```python
from build123d import *

# Parameters (mm, degrees)
SKETCH3_W           = 214
SKETCH3_H           = 93.282032303
BOSS_EXTRUDE1_DEPTH = 12.7
SKETCH2_R           = 9
CUT_EXTRUDE1_DEPTH  = 10
SKETCH5_R           = 7
CUT_EXTRUDE2_DEPTH  = 10


with BuildPart() as part:
    # Sketch3 → Boss-Extrude1 (new body)
    with BuildSketch(Plane(origin=(0, 0, 0), x_dir=(1, 0, 0), z_dir=(0, 1, 0))):
        with Locations((95, 34.641016152)):
            Rectangle(SKETCH3_W, SKETCH3_H)
    extrude(amount=BOSS_EXTRUDE1_DEPTH)

    # Sketch2 → Cut-Extrude1 (cut)
    with BuildSketch(Plane(origin=(0, 0, 0), x_dir=(1, 0, 0), z_dir=(0, 1, 0))):
        Circle(SKETCH2_R)
        with Locations((20, 0)):
            Circle(SKETCH2_R)
        with Locations((40, 0)):
            Circle(SKETCH2_R)
        with Locations((60, 0)):
            Circle(SKETCH2_R)
        with Locations((80, 0)):
            Circle(SKETCH2_R)
        with Locations((100, 0)):
            Circle(SKETCH2_R)
        with Locations((120, 0)):
            Circle(SKETCH2_R)
        with Locations((140, 0)):
            Circle(SKETCH2_R)
        with Locations((160, 0)):
            Circle(SKETCH2_R)
        with Locations((180, 0)):
            Circle(SKETCH2_R)
        with Locations((10, 17.320508076)):
            Circle(SKETCH2_R)
        with Locations((30, 17.320508076)):
            Circle(SKETCH2_R)
        with Locations((50, 17.320508076)):
            Circle(SKETCH2_R)
        with Locations((70, 17.320508076)):
            Circle(SKETCH2_R)
        with Locations((90, 17.320508076)):
            Circle(SKETCH2_R)
        with Locations((110, 17.320508076)):
            Circle(SKETCH2_R)
        with Locations((130, 17.320508076)):
            Circle(SKETCH2_R)
        with Locations((150, 17.320508076)):
            Circle(SKETCH2_R)
        with Locations((170, 17.320508076)):
            Circle(SKETCH2_R)
        with Locations((190, 17.320508076)):
            Circle(SKETCH2_R)
        with Locations((0, 34.641016151)):
            Circle(SKETCH2_R)
        with Locations((20, 34.641016151)):
            Circle(SKETCH2_R)
        with Locations((40, 34.641016151)):
            Circle(SKETCH2_R)
        with Locations((60, 34.641016151)):
            Circle(SKETCH2_R)
        with Locations((80, 34.641016151)):
            Circle(SKETCH2_R)
        with Locations((100, 34.641016151)):
            Circle(SKETCH2_R)
        with Locations((120, 34.641016151)):
            Circle(SKETCH2_R)
        with Locations((140, 34.641016151)):
            Circle(SKETCH2_R)
        with Locations((160, 34.641016151)):
            Circle(SKETCH2_R)
        with Locations((180, 34.641016151)):
            Circle(SKETCH2_R)
        with Locations((10, 51.961524227)):
            Circle(SKETCH2_R)
        with Locations((30, 51.961524227)):
            Circle(SKETCH2_R)
        with Locations((50, 51.961524227)):
            Circle(SKETCH2_R)
        with Locations((70, 51.961524227)):
            Circle(SKETCH2_R)
        with Locations((90, 51.961524227)):
            Circle(SKETCH2_R)
        with Locations((110, 51.961524227)):
            Circle(SKETCH2_R)
        with Locations((130, 51.961524227)):
            Circle(SKETCH2_R)
        with Locations((150, 51.961524227)):
            Circle(SKETCH2_R)
        with Locations((170, 51.961524227)):
            Circle(SKETCH2_R)
        with Locations((190, 51.961524227)):
            Circle(SKETCH2_R)
        with Locations((0, 69.282032303)):
            Circle(SKETCH2_R)
        with Locations((20, 69.282032303)):
            Circle(SKETCH2_R)
        with Locations((40, 69.282032303)):
            Circle(SKETCH2_R)
        with Locations((60, 69.282032303)):
            Circle(SKETCH2_R)
        with Locations((80, 69.282032303)):
            Circle(SKETCH2_R)
        with Locations((100, 69.282032303)):
            Circle(SKETCH2_R)
        with Locations((120, 69.282032303)):
            Circle(SKETCH2_R)
        with Locations((140, 69.282032303)):
            Circle(SKETCH2_R)
        with Locations((160, 69.282032303)):
            Circle(SKETCH2_R)
        with Locations((180, 69.282032303)):
            Circle(SKETCH2_R)
    extrude(amount=CUT_EXTRUDE1_DEPTH, mode=Mode.SUBTRACT)

    # Sketch5 → Cut-Extrude2 (cut)
    with BuildSketch(Plane.XZ.offset(-10)):
        Circle(SKETCH5_R)
        with Locations((20, 0)):
            Circle(SKETCH5_R)
        with Locations((40, 0)):
            Circle(SKETCH5_R)
        with Locations((80, 0)):
            Circle(SKETCH5_R)
        with Locations((60, 0)):
            Circle(SKETCH5_R)
        with Locations((100, 0)):
            Circle(SKETCH5_R)
        with Locations((120, 0)):
            Circle(SKETCH5_R)
        with Locations((140, 0)):
            Circle(SKETCH5_R)
        with Locations((160, 0)):
            Circle(SKETCH5_R)
        with Locations((180, 0)):
            Circle(SKETCH5_R)
        with Locations((190, -17.320508076)):
            Circle(SKETCH5_R)
        with Locations((170, -17.320508076)):
            Circle(SKETCH5_R)
        with Locations((150, -17.320508076)):
            Circle(SKETCH5_R)
        with Locations((130, -17.320508076)):
            Circle(SKETCH5_R)
        with Locations((110, -17.320508076)):
            Circle(SKETCH5_R)
        with Locations((90, -17.320508076)):
            Circle(SKETCH5_R)
        with Locations((70, -17.320508076)):
            Circle(SKETCH5_R)
        with Locations((50, -17.320508076)):
            Circle(SKETCH5_R)
        with Locations((30, -17.320508076)):
            Circle(SKETCH5_R)
        with Locations((10, -17.320508076)):
            Circle(SKETCH5_R)
        with Locations((0, -34.641016151)):
            Circle(SKETCH5_R)
        with Locations((20, -34.641016151)):
            Circle(SKETCH5_R)
        with Locations((40, -34.641016151)):
            Circle(SKETCH5_R)
        with Locations((60, -34.641016151)):
            Circle(SKETCH5_R)
        with Locations((80, -34.641016151)):
            Circle(SKETCH5_R)
        with Locations((100, -34.641016151)):
            Circle(SKETCH5_R)
        with Locations((120, -34.641016151)):
            Circle(SKETCH5_R)
        with Locations((140, -34.641016151)):
            Circle(SKETCH5_R)
        with Locations((160, -34.641016151)):
            Circle(SKETCH5_R)
        with Locations((180, -34.641016151)):
            Circle(SKETCH5_R)
        with Locations((190, -51.961524227)):
            Circle(SKETCH5_R)
        with Locations((170, -51.961524227)):
            Circle(SKETCH5_R)
        with Locations((150, -51.961524227)):
            Circle(SKETCH5_R)
        with Locations((130, -51.961524227)):
            Circle(SKETCH5_R)
        with Locations((110, -51.961524227)):
            Circle(SKETCH5_R)
        with Locations((90, -51.961524227)):
            Circle(SKETCH5_R)
        with Locations((70, -51.961524227)):
            Circle(SKETCH5_R)
        with Locations((50, -51.961524227)):
            Circle(SKETCH5_R)
        with Locations((30, -51.961524227)):
            Circle(SKETCH5_R)
        with Locations((10, -51.961524227)):
            Circle(SKETCH5_R)
        with Locations((20, -69.282032303)):
            Circle(SKETCH5_R)
        with Locations((40, -69.282032303)):
            Circle(SKETCH5_R)
        with Locations((60, -69.282032303)):
            Circle(SKETCH5_R)
        with Locations((80, -69.282032303)):
            Circle(SKETCH5_R)
        with Locations((100, -69.282032303)):
            Circle(SKETCH5_R)
        with Locations((120, -69.282032303)):
            Circle(SKETCH5_R)
        with Locations((140, -69.282032303)):
            Circle(SKETCH5_R)
        with Locations((160, -69.282032303)):
            Circle(SKETCH5_R)
        with Locations((180, -69.282032303)):
            Circle(SKETCH5_R)
        with Locations((0, -69.282032303)):
            Circle(SKETCH5_R)
    extrude(amount=-CUT_EXTRUDE2_DEPTH, mode=Mode.SUBTRACT)


solid = part.part
```
For this review, take the finished solid that the model builds, in its own axes (mm). A direction names the side the tool comes from. Coordinates: 2 decimals unless noted, no trailing zeros. Put each result on its own line as item: value.
1. For pin 1 (23.5 mm diameter, centred on x = 130, z = -17.32, fed in from +Y); pin 2 (9 mm diameter, centred on x = 152, z = -13.5, fed in from -Y), all flat-tipped, find the tip position at first contact; note any pin that passes through.
Values found:
pin 1: y = 12.7
pin 2: y = 10
2. Machinability: for faces 1 (the flat face through (190, 10, -44.7)), 2 (the cylindrical face through (13.763, 11.331, -11.418)), which of the approach directions +Z, -Z, +X, -X, +Y, -Y give a long, thin tool a straight path to every point of the face, cutting with its end or side? Answer none if there is none.
Values found:
face 1: -Y
face 2: +Y, -Y
3. Wall thickness on probe 1 along Z at (x, y) = (120, 11.8); probe 2 along Z at (x, y) = (30, 5.5); probe 3 along Z at (x, y) = (0, 4): over which ranges is each line inside the solid? List them lowest first.
Values found:
probe 1: -81.28 to -76.28, -62.28 to -41.64, -27.64 to -7, 7 to 12
probe 2: -81.28 to -60.96, -42.96 to -26.32, -8.32 to 12
probe 3: -81.28 to -78.28, -60.28 to -43.64, -25.64 to -9, 9 to 12
4. Add section A-A, the plane z = 0. Count the separate pieces of the cut face and the enclosed holes in it, then the cut area to 3 significant figures.
Values found:
separate pieces: 11
enclosed holes: 0
area: 540 mm²
